Check sheet for the modelled part. Datum: model origin and axes. Units: mm. A direction names the side the tool comes from. Give positions to 0.01 mm unless a question says otherwise; leave off trailing zeros. Loops run counter-clockwise (first coordinate to the right, second up) from the corner with the lowest first, then second, coordinate; pieces in that order, holes last. Notation, with made-up numbers: (85.25, 76.25) - (96.25, 76.25) arc R10 cw to (96.25, 82.25) - close; hole circle Ø8 at (-30.75, 7). An arc over 180 degrees is marked (long way). Answer in a Markdown table with one row per item. Add a question column.
(1) Sectioned sample at B-B on y = 11. Enter the section's corners in (x, z).
(2) Set-up check for faces 4 (the face through (-6, 10, -3)), 5 (the face through (-3.6, 6, -3)), 6 (the face through (-7.6, 6, -3)): record each of +Z, -Z, +X, -X, +Y, -Y from which the full face is reachable in a straight line by a thin tool's end or side.
(3) Go/stop test with flat-tipped pins: P1, Ø2, axis at y = 7.5, z = -5, coming from the -X side; P2, Ø4, axis at x = -39.1, y = 2, coming from the +Z side; P3, Ø3, axis at x = -6, z = -4, coming from the -Y side; P4, Ø4, axis at x = -26.5, y = 7.5, coming from the -Z side. Record where each tip stops, or that it passes through.
(4) Sectioned sample at A-A on x = -1.9. Enter the section's corners in (y, z), then the cut area to 3 significant figures.
(5) Thickness scan on L1, parallel to Y at x = -1.9, z = 1.15; L2, parallel to Z at x = -34, y = 2; L3, parallel to X at y = 5.25, z = -3. Record the ranges inside material, lowest first.
(6) Draft check along X on faces 1 (the face through (0, 6, 1)), 2 (the face through (-0.514, 1.425, 1.521)), 3 (the face through (-6, 3, -3)). Enter one of: released by +X, released by -X, zero draft, split by the parting line, or undercut.
(7) Sectioned sample at C-C on y = 6. Enter the section's corners in (x, z), then the cut area to 3 significant figures.
(8) Sectioned sample at D-D on z = -3.25. Enter the section's corners in (x, y).
from build123d import *

# Parameters (mm, degrees)
CROQUIS1_W              = 41
CROQUIS1_H              = 13
SALIENTE_EXTRUIR1_DEPTH = 3
CROQUIS2_R              = 1.5
CORTAR_EXTRUIR1_DEPTH   = 44.116122275
CROQUIS3_W              = 4
CROQUIS3_H              = 7
SALIENTE_EXTRUIR2_DEPTH = 7


with BuildPart() as part:
    # Croquis1 → Saliente-Extruir1 (new body)
    with BuildSketch(Plane.XY):
        with Locations((-20.5, 6.5)):
            Rectangle(CROQUIS1_W, CROQUIS1_H)
    extrude(amount=SALIENTE_EXTRUIR1_DEPTH)

    # Croquis2 → Cortar-Extruir1 (cut, through all)
    with BuildSketch(Plane.XY.offset(3)):
        with Locations((-1.9, 11)):
            Circle(CROQUIS2_R)
        with Locations((-1.9, 2)):
            Circle(CROQUIS2_R)
        with Locations((-39.1, 11)):
            Circle(CROQUIS2_R)
        with Locations((-39.1, 2)):
            Circle(CROQUIS2_R)
    extrude(amount=-CORTAR_EXTRUIR1_DEPTH, mode=Mode.SUBTRACT)

    # Croquis3 → Saliente-Extruir2 (add)
    with BuildSketch(Plane(origin=(0, 0, 0), x_dir=(-1, 0, 0), z_dir=(0, 0, -1))):
        with Locations((5.6, 6.5)):
            Rectangle(CROQUIS3_W, CROQUIS3_H)
    extrude(amount=SALIENTE_EXTRUIR2_DEPTH)


solid = part.part
Reply:
| question | item | result |
|---|---|---|
| 1 | outline | (-41, 0) - (-40.6, 0) - (-40.6, 3) - (-41, 3) - close; (-37.6, 0) - (-3.4, 0) - (-3.4, 3) - (-37.6, 3) - close; (-0.4, 0) - (0, 0) - (0, 3) - (-0.4, 3) - close |
| 2 | face 4 | -Z, +X, -X, +Y |
| 2 | face 5 | -Z, +X, +Y, -Y |
| 2 | face 6 | -Z, -X, +Y, -Y |
| 3 | P1 | x = -7.6 |
| 3 | P2 | z = 3 |
| 3 | P3 | y = 3 |
| 3 | P4 | z = 0 |
| 4 | outline | (0, 0) - (0.5, 0) - (0.5, 3) - (0, 3) - close; (3.5, 0) - (9.5, 0) - (9.5, 3) - (3.5, 3) - close; (12.5, 0) - (13, 0) - (13, 3) - (12.5, 3) - close |
| 4 | area | 21.0 mm^2 |
| 5 | L1 | 0 to 0.5, 3.5 to 9.5, 12.5 to 13 |
| 5 | L2 | 0 to 3 |
| 5 | L3 | -7.6 to -3.6 |
| 6 | face 1 | released by +X |
| 6 | face 2 | undercut |
| 6 | face 3 | zero draft |
| 7 | outline | (-41, 0) - (-7.6, 0) - (-7.6, -7) - (-3.6, -7) - (-3.6, 0) - (0, 0) - (0, 3) - (-41, 3) - close |
| 7 | area | 151 mm^2 |
| 8 | outline | (-7.6, 3) - (-3.6, 3) - (-3.6, 10) - (-7.6, 10) - close |
